Geometry: see drawing. Coordinates: mm, zero at the bounding-box minimum. Give positions to 0.01 mm unless a question says otherwise; leave off trailing zeros. Loops run counter-clockwise (first coordinate to the right, second up) from the corner with the lowest first, then second, coordinate; pieces in that order, holes last. Notation, with made-up numbers: M -12,52.5 L 12,52.5 A25 ccw 12,89.5 Z; hole C 45,76.25 d4. An arc over 180 degrees is marked long. Put each result on its own line as item: value.
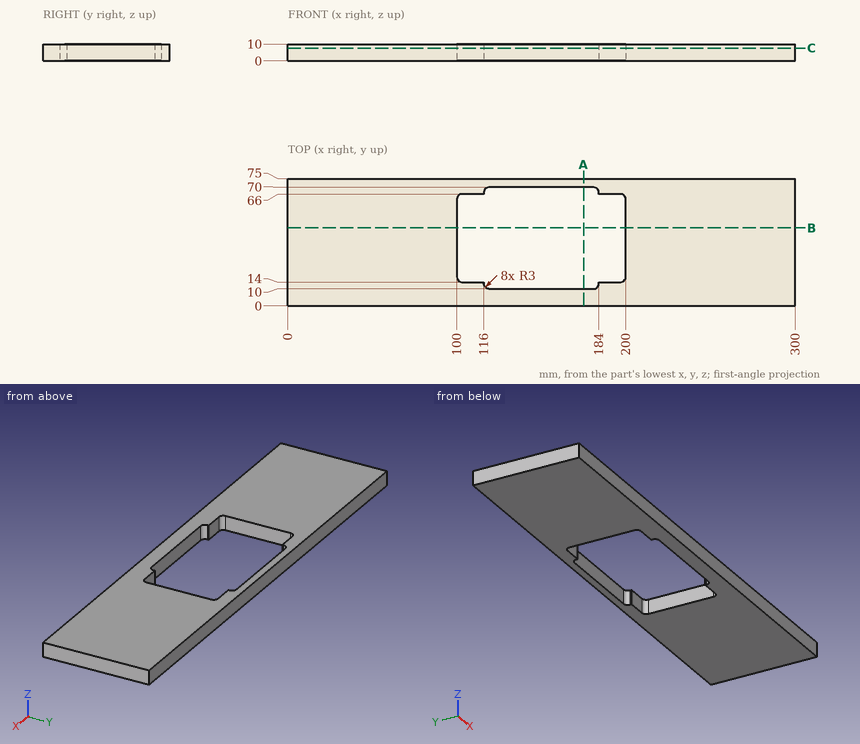
Item 1: Line query: probe 1 along X at (y, z) = (18, 6.25); probe 2 along Y at (x, z) = (189, 4.5); probe 3 along Y at (x, z) = (171.5, 7.5). Output: solid intervals per line, ascending. Write a range as [from, to].
Output values:
probe 1: [0, 100], [200, 300]
probe 2: [0, 14], [66, 75]
probe 3: [0, 10], [70, 75]
Item 2: Section B-B on y = 46. Output: boundary loops of the cut face in (x, z).
Output values:
outline: M 0,0 L 100,0 L 100,10 L 0,10 Z; M 200,0 L 300,0 L 300,10 L 200,10 Z
Item 3: Section C-C on z = 7.5. Output: boundary loops of the cut face in (x, y).
Output values:
outline: M 0,0 L 300,0 L 300,75 L 0,75 Z; hole M 100,17 A3 ccw 103,14 L 116,14 L 116,13 A3 ccw 119,10 L 181,10 A3 ccw 184,13 L 184,14 L 197,14 A3 ccw 200,17 L 200,63 A3 ccw 197,66 L 184,66 L 184,67 A3 ccw 181,70 L 119,70 A3 ccw 116,67 L 116,66 L 103,66 A3 ccw 100,63 Z
Item 4: Section A-A on x = 175. Output: boundary loops of the cut face in (y, z).
Output values:
outline: M 0,0 L 10,0 L 10,10 L 0,10 Z; M 70,0 L 75,0 L 75,10 L 70,10 Z
